```python
from build123d import *

# Parameters (mm, degrees)
SKETCH004_R          = 1.475
SKETCH004_R_2        = 10
PAD003_DEPTH         = 10
SKETCH009_R          = 2.76
POCKET002_DEPTH      = 3
SKETCH014_R          = 11.1
POCKET006_DEPTH      = 2
SKETCH016_W          = 21.25
SKETCH016_H          = 3
POCKET_DEPTH         = 21.001
SKETCH015_R          = 1.5
POCKET007_DEPTH      = 21.001
POCKET007_DEPTH_BACK = 21.001
SKETCH_R             = 2.5
POCKET008_DEPTH      = 3
SKETCH017_R          = 4.09
POCKET009_DEPTH      = 0.001
POCKET009_DEPTH_BACK = 10.001
SKETCH018_R          = 4.09
SKETCH018_W          = 2.5
SKETCH018_H          = 5.73
PAD_DEPTH            = 10
SKETCH019_W          = 5.73
SKETCH019_H          = 2.5
POCKET010_DEPTH      = 0.001
POCKET010_DEPTH_BACK = 10.001
SKETCH020_R          = 1.5
POCKET011_DEPTH      = 12
SKETCH045_R          = 1.5
POCKET027_DEPTH      = 5
SKETCH046_R          = 1.5
POCKET028_DEPTH      = 5
SKETCH052_W          = 22.5
SKETCH052_H          = 0.2
POCKET034_DEPTH      = 0.001
POCKET034_DEPTH_BACK = 10.001


with BuildPart() as part:
    # Sketch004 → Pad003 (new body)
    with BuildSketch(Plane.XY):
        Polygon((-21, 21), (21, 21), (21, 10), (21, -10), (21, -21), (21, -44.75), (14.9, -44.75), (14.9, -21), (-7.6, -21), (-7.6, -44.75), (-14.6, -44.75), (-14.6, -21), (-21, -21), align=None)
        with Locations((-15.5, 15.5)):
            Circle(SKETCH004_R, mode=Mode.SUBTRACT)
        with Locations((15.5, 15.5)):
            Circle(SKETCH004_R, mode=Mode.SUBTRACT)
        with Locations((-15.5, -15.5)):
            Circle(SKETCH004_R, mode=Mode.SUBTRACT)
        with Locations((15.5, -15.5)):
            Circle(SKETCH004_R, mode=Mode.SUBTRACT)
        with Locations((0, 15.5)):
            Circle(SKETCH004_R, mode=Mode.SUBTRACT)
        with Locations((0, -15.5)):
            Circle(SKETCH004_R, mode=Mode.SUBTRACT)
        Circle(SKETCH004_R_2, mode=Mode.SUBTRACT)
    extrude(amount=PAD003_DEPTH)

    # Sketch009 → Pocket002 (cut)
    with BuildSketch(Plane.XY):
        with Locations((-15.5, 15.5)):
            Circle(SKETCH009_R)
        with Locations((15.5, 15.5)):
            Circle(SKETCH009_R)
        with Locations((-15.5, -15.5)):
            Circle(SKETCH009_R)
        with Locations((15.5, -15.5)):
            Circle(SKETCH009_R)
        with Locations((0, 15.5)):
            Circle(SKETCH009_R)
        with Locations((0, -15.5)):
            Circle(SKETCH009_R)
    extrude(amount=POCKET002_DEPTH, mode=Mode.SUBTRACT)

    # Sketch014 (on Face5 of Pocket002) → Pocket006 (cut)
    with BuildSketch(Plane.XY.offset(10)):
        Circle(SKETCH014_R)
    extrude(amount=-POCKET006_DEPTH, mode=Mode.SUBTRACT)

    # Sketch016 → Pocket (cut, through all)
    with BuildSketch(Plane.YZ):
        with Locations((-34.125, 10.1)):
            Rectangle(SKETCH016_W, SKETCH016_H)
    extrude(amount=POCKET_DEPTH, mode=Mode.SUBTRACT)

    # Sketch015 → Pocket007 (cut, two sides)
    with BuildSketch(Plane.YZ) as pocket007_sk:
        with Locations((-39.85, 4.3)):
            Circle(SKETCH015_R)
        with Locations((-29.85, 4.3)):
            Circle(SKETCH015_R)
    extrude(amount=-POCKET007_DEPTH, mode=Mode.SUBTRACT)
    extrude(pocket007_sk.sketch, amount=POCKET007_DEPTH_BACK, mode=Mode.SUBTRACT)

    # Sketch (on DatumPlane) → Pocket008 (cut)
    with BuildSketch(Plane.YZ.offset(21)):
        with Locations((-39.85, 4.3)):
            Circle(SKETCH_R)
        with Locations((-29.85, 4.3)):
            Circle(SKETCH_R)
    extrude(amount=-POCKET008_DEPTH, mode=Mode.SUBTRACT)

    # Sketch017 → Pocket009 (cut, two sides)
    with BuildSketch(Plane.XY) as pocket009_sk:
        with Locations((-18.5, 0)):
            Circle(SKETCH017_R)
        with Locations((18.5, 0)):
            Circle(SKETCH017_R)
    extrude(amount=-POCKET009_DEPTH, mode=Mode.SUBTRACT)
    extrude(pocket009_sk.sketch, amount=POCKET009_DEPTH_BACK, mode=Mode.SUBTRACT)

    # Sketch018 → Pad (join)
    with BuildSketch(Plane.XY):
        with BuildLine():
            ThreePointArc((-21, 10.7688), (-29.555182, 0), (-21, -10.7688))
            Line((-13.41, -10.7688), (-21, -10.7688))
            Line((-13.41, 10.7688), (-13.41, -10.7688))
            Line((-21, 10.7688), (-13.41, 10.7688))
        make_face()
        with Locations((-18.5, 0)):
            Circle(SKETCH018_R, mode=Mode.SUBTRACT)
        with Locations((-25.84, 0)):
            Rectangle(SKETCH018_W, SKETCH018_H, mode=Mode.SUBTRACT)
        with BuildLine():
            ThreePointArc((21, -10.7688), (29.555182, 0), (21, 10.7688))
            Line((13.41, 10.7688), (21, 10.7688))
            Line((13.41, 10.7688), (13.41, -10.7688))
            Line((13.41, -10.7688), (21, -10.7688))
        make_face()
        with Locations((18.5, 0)):
            Circle(SKETCH018_R, mode=Mode.SUBTRACT)
        with Locations((25.84, 0)):
            Rectangle(SKETCH018_W, SKETCH018_H, mode=Mode.SUBTRACT)
    extrude(amount=PAD_DEPTH)

    # Sketch019 → Pocket010 (cut, two sides)
    with BuildSketch(Plane.XY) as pocket010_sk:
        with Locations((-7.5, 16.75)):
            Rectangle(SKETCH019_W, SKETCH019_H)
        with Locations((7.5, 16.75)):
            Rectangle(SKETCH019_W, SKETCH019_H)
    extrude(amount=-POCKET010_DEPTH, mode=Mode.SUBTRACT)
    extrude(pocket010_sk.sketch, amount=POCKET010_DEPTH_BACK, mode=Mode.SUBTRACT)

    # Sketch020 (on DatumPlane) → Pocket011 (cut)
    with BuildSketch(Plane(origin=(0, 21, 0), x_dir=(-1, 0, 0), z_dir=(0, 1, 0))):
        with Locations((-7.5, 5)):
            Circle(SKETCH020_R)
        with Locations((7.5, 5)):
            Circle(SKETCH020_R)
    extrude(amount=-POCKET011_DEPTH, mode=Mode.SUBTRACT)

    # Sketch045 (on DatumPlane) → Pocket027 (cut, symmetric)
    with BuildSketch(Plane.YZ.offset(24.59)):
        with Locations((0, 5)):
            Circle(SKETCH045_R)
    extrude(amount=POCKET027_DEPTH, both=True, mode=Mode.SUBTRACT)

    # Sketch046 (on DatumPlane) → Pocket028 (cut, symmetric)
    with BuildSketch(Plane(origin=(-24.59, 0, 0), x_dir=(0, -1, 0), z_dir=(-1, 0, 0))):
        with Locations((0, 5)):
            Circle(SKETCH046_R)
    extrude(amount=POCKET028_DEPTH, both=True, mode=Mode.SUBTRACT)

    # Sketch052 → Pocket034 (cut, two sides)
    with BuildSketch(Plane.XY) as pocket034_sk:
        with Locations((3.65, -20.9)):
            Rectangle(SKETCH052_W, SKETCH052_H)
    extrude(amount=-POCKET034_DEPTH, mode=Mode.SUBTRACT)
    extrude(pocket034_sk.sketch, amount=POCKET034_DEPTH_BACK, mode=Mode.SUBTRACT)


with BuildPart() as part_1:
    # Body003 placement: moved
    add(part.part.moved(Location((0, 0, 40))))


solid = part_1.part
```
The listing builds one solid part. Answer for the finished solid, in the listing's coordinates (mm). A direction names the side the tool comes from. Coordinates: 2 decimals unless noted, no trailing zeros. Write each loop counter-clockwise with the first axis right and the second up, starting at its lowest first coordinate (ties: lowest second). Pieces come first, ordered by that corner, then holes. Notation, with made-up numbers: (28, -39) - (39, -39) arc R11 ccw to (39, -29) - close; hole circle Ø8 at (82.5, 46.25). An arc over 180 degrees is marked (long way). Return JSON: item names as keys, results as strings. Group by question number.
1. Which of the six approach directions +Z, -Z, +X, -X, +Y, -Y give full straight-line access (tool end or side, diameter ignored) to faces 5 (the flat face through (-6, 15.5, 44)), 6 (the flat face through (-7, 9, 45)), 7 (the flat face through (-14, -17, 43)), 8 (the flat face through (-0.4, -11.4, 50))?
2. A cutting plane is placed at C-C, the plane y = 5. Determine the outline of the cut face in (x, z), plus the area to 3 significant figures.
3. A cutting plane is placed at D-D, the plane x = 7.5. Determine the outline of the cut face in (y, z).
4. Straight lines are drawn through the part: L1, parallel to X at y = -15.5, z = 46.75 (3 decimals); L2, parallel to X at y = -27, z = 41.25; L3, parallel to Y at x = 0, z = 46 (3 decimals). For each, find the intervals that lie inside material, in ascending order.
5. Given pin 1 (4.5 mm diameter, centred on y = 1, z = 46.5, fed in from -X); pin 2 (1.2 mm diameter, centred on y = 17, z = 43, fed in from +X); pin 3 (3 mm diameter, centred on x = -25.5, z = 45, fed in from -Y); pin 4 (2 mm diameter, centred on y = -5.5, z = 42, fed in from -X), each flat-ended and moving along its own axis, determine where each tip first touches the part or whether it passes through.
6. Determine the mould class of faces 1 (the flat face through (-18, -21, 45)), 2 (the cylindrical face through (-14.093, 15.943, 46.451)), 3 (the flat face through (18, -34, 48.6)), 4 (the flat face through (27.09, 1.2, 43.8)) for opening direction Y: released by +Y, released by -Y, zero draft, split by the parting line, or undercut.
7. A cutting plane is placed at B-B, the plane x = 19.5. Determine the outline of the cut face in (y, z), plus the area to 3 significant figures.
8. A cutting plane is placed at A-A, the plane y = -39.85. Determine the outline of the cut face in (x, z).
Ans:
{
 "1": {"face 5": "+Z, -Z", "face 6": "+Y", "face 7": "-Z", "face 8": "+Z, +X, -X, +Y, -Y"},
 "2": {"outline": "(-28.36, 40) - (-8.66, 40) - (-8.66, 48) - (-9.91, 48) - (-9.91, 50) - (-28.36, 50) - close; (8.66, 40) - (28.36, 40) - (28.36, 50) - (9.91, 50) - (9.91, 48) - (8.66, 48) - close", "area": "389 mm²"},
 "3": {"outline": "(-20.8, 40) - (-6.61, 40) - (-6.61, 48) - (-8.18, 48) - (-8.18, 50) - (-20.8, 50) - close; (6.61, 40) - (15.5, 40) - (15.5, 43.5) - (9, 43.5) - (9, 46.5) - (15.5, 46.5) - (15.5, 50) - (8.18, 50) - (8.18, 48) - (6.61, 48) - close; (18, 40) - (21, 40) - (21, 43.5) - (18, 43.5) - close; (18, 46.5) - (21, 46.5) - (21, 50) - (18, 50) - close"},
 "4": {"L1": "-21 to -16.975, -14.025 to -1.475, 1.475 to 14.025, 16.975 to 21", "L2": "-14.6 to -7.6, 14.9 to 21", "L3": "-20.8 to -16.975, -14.025 to -10, 10 to 14.025, 16.975 to 21"},
 "5": {"pin 1": "x = -29.56", "pin 2": "x = 21", "pin 3": "y = -9.59", "pin 4": "x = -28.6"},
 "6": {"face 1": "released by -Y", "face 2": "undercut", "face 3": "zero draft", "face 4": "undercut"},
 "7": {"outline": "(-44.75, 40) - (-3.97, 40) - (-3.97, 50) - (-23.5, 50) - (-23.5, 48.6) - (-44.75, 48.6) - close; (3.97, 40) - (21, 40) - (21, 50) - (3.97, 50) - close; hole circle Ø5 at (-39.85, 44.3); hole circle Ø5 at (-29.85, 44.3)", "area": "509 mm²"},
 "8": {"outline": "(-14.6, 40) - (-7.6, 40) - (-7.6, 42.8) - (-14.6, 42.8) - close; (-14.6, 45.8) - (-7.6, 45.8) - (-7.6, 50) - (-14.6, 50) - close; (14.9, 40) - (21, 40) - (21, 41.8) - (18, 41.8) - (18, 42.8) - (14.9, 42.8) - close; (14.9, 45.8) - (18, 45.8) - (18, 46.8) - (21, 46.8) - (21, 48.6) - (14.9, 48.6) - close"}
}
